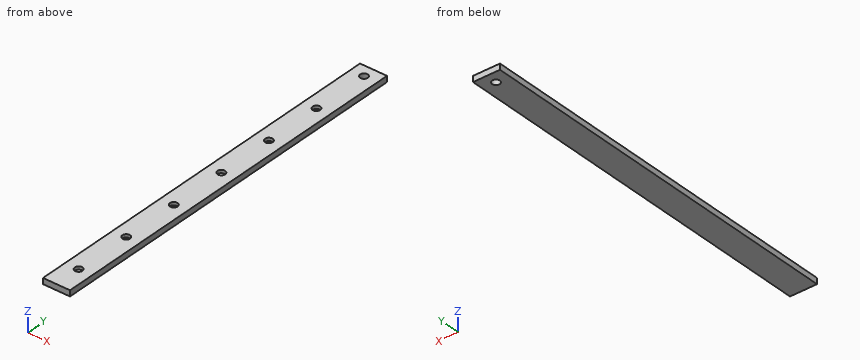
from build123d import *

# Parameters (mm, degrees)
SKETCH1_W           = 70
SKETCH1_H           = 15
BOSS_EXTRUDE1_DEPTH = 1000
SKETCH2_R           = 10
CUT_EXTRUDE1_DEPTH  = 15
SKETCH3_R           = 10
CUT_EXTRUDE2_DEPTH  = 8


with BuildPart() as part:
    # Sketch1 → Boss-Extrude1 (new body)
    with BuildSketch(Plane(origin=(0, 0, 0), x_dir=(1, 0, 0), z_dir=(0, 1, 0))):
        with Locations((-35, -7.5)):
            Rectangle(SKETCH1_W, SKETCH1_H)
    extrude(amount=BOSS_EXTRUDE1_DEPTH)

    # Sketch2 → Cut-Extrude1 (cut)
    with BuildSketch(Plane.XY.offset(15)):
        with Locations((-35, 970)):
            Circle(SKETCH2_R)
    extrude(amount=-CUT_EXTRUDE1_DEPTH, mode=Mode.SUBTRACT)

    # Sketch3 → Cut-Extrude2 (cut)
    with BuildSketch(Plane.XY.offset(15)):
        with Locations((-35, 820)):
            Circle(SKETCH3_R)
        with Locations((-35, 670)):
            Circle(SKETCH3_R)
        with Locations((-35, 520)):
            Circle(SKETCH3_R)
        with Locations((-35, 370)):
            Circle(SKETCH3_R)
        with Locations((-35, 220)):
            Circle(SKETCH3_R)
        with Locations((-35, 70)):
            Circle(SKETCH3_R)
    extrude(amount=-CUT_EXTRUDE2_DEPTH, mode=Mode.SUBTRACT)


solid = part.part
Input: part model. Units: mm. Frame: model coordinates. Coordinates: 2 decimals unless noted, no trailing zeros. Loops run counter-clockwise (first coordinate to the right, second up) from the corner with the lowest first, then second, coordinate; pieces in that order, holes last.
Q1. Cut plane A-A (y = 970). Output: boundary loops of the cut face in (x, z), then the cut area to 3 significant figures.
Q2. Cut plane B-B (y = 370). Output: boundary loops of the cut face in (x, z).
Q3. Contact query for a flat-ended pin moving along its axis: pin 1 (10 mm diameter, centred on x = -34, y = 65.5, fed in from +Z). Output: stop coordinate, or through.
Q4. Material intervals for line 1 (X direction, y = 670, z = 8.75); line 2 (Y direction, x = -28, z = 4.25), sorted ascending.
Working result:
1. outline: (-70, 0) - (-45, 0) - (-45, 15) - (-70, 15) - close; (-25, 0) - (0, 0) - (0, 15) - (-25, 15) - close
1. area: 750 mm2
2. outline: (-70, 0) - (0, 0) - (0, 15) - (-25, 15) - (-25, 7) - (-45, 7) - (-45, 15) - (-70, 15) - close
3. pin 1: stops at z = 7
4. line 1: x = -70 to -45, -25 to 0
4. line 2: y = 0 to 962.86, 977.14 to 1000
